```python
from build123d import *

# Parameters (mm, degrees)
CROQUIS1_W              = 50
CROQUIS1_H              = 50
CROQUIS1_W_2            = 47.6
CROQUIS1_H_2            = 47.6
SALIENTE_EXTRUIR1_DEPTH = 300
CROQUIS2_R              = 2.5
CORTAR_EXTRUIR1_DEPTH   = 306.163890393
CROQUIS3_R              = 4.5
CORTAR_EXTRUIR2_DEPTH   = 306.163890393
CROQUIS4_R              = 8
CORTAR_EXTRUIR3_DEPTH   = 2
CROQUIS5_R              = 2.5
CORTAR_EXTRUIR4_DEPTH   = 306.163890393


with BuildPart() as part:
    # Croquis1 → Saliente-Extruir1 (new body)
    with BuildSketch(Plane.XY):
        Rectangle(CROQUIS1_W, CROQUIS1_H)
        Rectangle(CROQUIS1_W_2, CROQUIS1_H_2, mode=Mode.SUBTRACT)
    extrude(amount=SALIENTE_EXTRUIR1_DEPTH)

    # Croquis2 → Cortar-Extruir1 (cut, through all)
    with BuildSketch(Plane(origin=(25, 0, 0), x_dir=(0, 0, -1), z_dir=(1, 0, 0))):
        with Locations(Location((-295, 17.8, 0), (0, 0, 90))):
            Circle(CROQUIS2_R)
        with Locations(Location((-265, 17.8, 0), (0, 0, 90))):
            Circle(CROQUIS2_R)
        with Locations(Location((-265, -17.8, 0), (0, 0, 90))):
            Circle(CROQUIS2_R)
        with Locations(Location((-295, -17.8, 0), (0, 0, 90))):
            Circle(CROQUIS2_R)
    extrude(amount=-CORTAR_EXTRUIR1_DEPTH, mode=Mode.SUBTRACT)

    # Croquis3 → Cortar-Extruir2 (cut, through all)
    with BuildSketch(Plane(origin=(0, 25, 0), x_dir=(1, 0, 0), z_dir=(0, 1, 0))):
        with Locations(Location((0, -280, 0), (0, 0, 270))):
            Circle(CROQUIS3_R)
    extrude(amount=-CORTAR_EXTRUIR2_DEPTH, mode=Mode.SUBTRACT)

    # Croquis4 → Cortar-Extruir3 (cut)
    with BuildSketch(Plane.XZ.offset(25)):
        with Locations(Location((0, 30, 0), (0, 0, 270))):
            Circle(CROQUIS4_R)
    extrude(amount=-CORTAR_EXTRUIR3_DEPTH, mode=Mode.SUBTRACT)

    # Croquis5 → Cortar-Extruir4 (cut, through all)
    with BuildSketch(Plane.XZ.offset(25)):
        with Locations(Location((-18, 8, 0), (0, 0, 270))):
            Circle(CROQUIS5_R)
        with Locations(Location((-12, 54, 0), (0, 0, 270))):
            Circle(CROQUIS5_R)
        with Locations(Location((18, 8, 0), (0, 0, 90))):
            Circle(CROQUIS5_R)
        with Locations(Location((12, 54, 0), (0, 0, 90))):
            Circle(CROQUIS5_R)
    extrude(amount=-CORTAR_EXTRUIR4_DEPTH, mode=Mode.SUBTRACT)


solid = part.part
```
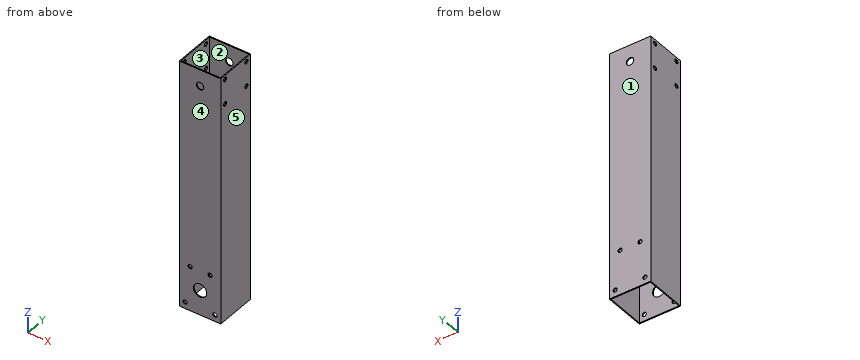
Design review of the part built by this model. Coordinates are the model's own, in mm. Face numbers are marked on the shaded views. A direction names the side the tool comes from. Round coordinates to 2 decimals unless told otherwise and drop trailing zeros. Write each loop counter-clockwise with the first axis right and the second up, starting at its lowest first coordinate (ties: lowest second). Pieces come first, ordered by that corner, then holes.
Item 1: For probe 1 along Z at (x, y) = (-24.5, -17.8); probe 2 along Y at (x, z) = (-24.6, 295); probe 3 along X at (y, z) = (-24.5, 54), list the stretches that pass through material, from the lowest coordinate up.
Item 2: The part is to be moulded in two halves that separate along X. For the marked faces 3, 4 and 5, say which applies: +X half, -X half, draft (parallel to the pull), parting line (faces both ways), or undercut.
Item 3: Clearance check with a flat-ended pin moving along its axis: pin 1 Ø3 at (x, z) = (-18, 8) entering from -Y. State where the tip first meets the part, or that it passes through.
Item 4: For the marked faces 1 and 2, list the 3-axis set-ups (+Z, -Z, +X, -X, +Y, -Y) from which the entire face can be reached by the end or side of a thin tool; tool diameter is ignored.
Item 5: We need section B-B on z = 54. Write out the cut boundary in (x, y).
Item 6: We need section D-D on z = 248.5. Write out the cut boundary in (x, y), and give its area (3 significant figures).
Item 7: We need section C-C on y = 4.5. Write out the cut boundary in (x, z).
Item 8: We need section A-A on x = 18. Write out the cut boundary in (y, z), and give its area (3 significant figures).
Returned:
1. probe 1: z = 0 to 262.5, 267.5 to 292.5, 297.5 to 300
1. probe 2: y = -25 to -20.3, -15.3 to 15.3, 20.3 to 25
1. probe 3: x = -25 to -14.5, -9.5 to 9.5, 14.5 to 25
2. face 3: undercut
2. face 4: draft
2. face 5: +X half
3. pin 1: passes through
4. face 1: +Z, -Z, +X, -X, +Y
4. face 2: +Z, -Z
5. outline: (-25, -25) - (-14.5, -25) - (-14.5, -23.8) - (-23.8, -23.8) - (-23.8, 23.8) - (-14.5, 23.8) - (-14.5, 25) - (-25, 25) - close; (-9.5, -25) - (9.5, -25) - (9.5, -23.8) - (-9.5, -23.8) - close; (-9.5, 23.8) - (9.5, 23.8) - (9.5, 25) - (-9.5, 25) - close; (14.5, -25) - (25, -25) - (25, 25) - (14.5, 25) - (14.5, 23.8) - (23.8, 23.8) - (23.8, -23.8) - (14.5, -23.8) - close
6. outline: (-25, -25) - (25, -25) - (25, 25) - (-25, 25) - close; hole (-23.8, -23.8) - (23.8, -23.8) - (23.8, 23.8) - (-23.8, 23.8) - close
6. area: 234 mm2
7. outline: (-25, 0) - (-23.8, 0) - (-23.8, 300) - (-25, 300) - close; (23.8, 0) - (25, 0) - (25, 300) - (23.8, 300) - close
8. outline: (-25, 0) - (-23.8, 0) - (-23.8, 5.5) - (-25, 5.5) - close; (-25, 10.5) - (-23.8, 10.5) - (-23.8, 300) - (-25, 300) - close; (23.8, 0) - (25, 0) - (25, 5.5) - (23.8, 5.5) - close; (23.8, 10.5) - (25, 10.5) - (25, 300) - (23.8, 300) - close
8. area: 708 mm2
